Autodesk Inventor part; units mm, degrees
ref_plane "YZ Plane" through (0, 0, 0) normal (1, 0, 0) x (0, 1, 0)
ref_plane "XZ Plane" through (0, 0, 0) normal (0, 1, 0) x (-1, 0, 0)
ref_plane "XY Plane" through (0, 0, 0) normal (0, 0, 1) x (1, 0, 0)
sketch "Sketch1" plane through (0, 0, 0) normal (0, 1, 0) x (-1, 0, 0)
  line L0 (606, 0) -> (606, -30)
  arc A0 (552, -118.7919) -> (606, -30) centre (506, -30) ccw
  arc A1 (0, -253.2892) -> (552, -118.7919) centre (0, 946.7108) ccw
  line L1 (0, 191.6842) -> (0, -191.6842)
  arc A2 (0, -247.2892) -> (549.24, -113.4644) centre (0, 946.7108) ccw
  arc A3 (549.24, -113.4644) -> (600, -30) centre (506, -30) ccw
  line L2 (600, -30) -> (600, 0)
  line L3 (600, 0) -> (606, 0)
  line L4 (0, -247.2892) -> (0, -253.2892)
  point P0 (0, 0)
  point P1 (0, 0)
  point P2 (0, -250.2892)
  point P3 (0, -163.7009)
  point P4 (0, -169.7009)
  dimension "d0" = 100
  dimension "d1" = 30
  dimension "d3" = 1200
  dimension "d6" = 6
  dimension "d11" = 1200
  dimension "d12" = 253.2892
revolve "Revolution1" add sketch "Sketch1" angle 360 about axis through (0, 0, 191.6842) along (0, 0, -1)
sketch "Sketch2" plane through (0, 0, 0) normal (0, 0, 1) x (1, 0, 0)
  circle A0 centre (0, 0) radius 16.75
  dimension "d8" = 33.5
extrude "Extrusion1" cut sketch "Sketch2" against normal through all
equation "\"d3\" = d11"
equation "\"Disherd_head_hight\" = d12"
properties part number "PNV - 704 dished head D1200" material "Steel"
Geometry check sheet. Reference: the model listing, model coordinates, mm. Coordinates: 2 decimals unless noted, no trailing zeros. One line per item, written item: value. Start each with the question number.
(1) Scan lines: line 1 along Y through (x, z) = (0, -20.75); line 2 along Y through (x, z) = (67.5, -34.5); line 3 along X through (y, z) = (453, -99.5). Record each from-to range of solid material in increasing order. Write a range as [from, to].
(2) Release check for a two-part mould opening along X. For faces 1 (the face through (-3.63, -16.35, -250.13)), 2 (the face through (586, 137, 0)), 3 (the face through (78.108, -594.894, -14.79)), 4 (the face through (605.414, 26.645, -15.21)) record: released by +X, released by -X, zero draft, split by the parting line, or undercut.
(3) Depth check by flat-ended pin: pin 1 (4 mm diameter, centred on x = 450.5, z = -91, fed in from +Y); pin 2 (10 mm diameter, centred on x = 297, y = 250.5, fed in from +Z); pin 3 (6 mm diameter, centred on y = 286.5, z = -83.5, fed in from -X). Enter the tip coordinate at first touch or a pass-through.
Filled sheet:
1. line 1: [-606, -600], [600, 606]
1. line 2: [-602.13, -596.08], [596.08, 602.13]
1. line 3: [-358.83, -344.79], [344.79, 358.83]
2. face 1: undercut
2. face 2: zero draft
2. face 3: undercut
2. face 4: split by the parting line
3. pin 1: y = 376.94
3. pin 2: z = -180.57
3. pin 3: x = -519
